from build123d import *

# Parameters (mm, degrees)
SKETCH1_R               = 25.65
SKETCH1_R_2             = 1.45
BOSS_EXTRUDE1_DEPTH     = 10
CUT_EXTRUDE2_DEPTH      = 38.627715849
CUT_EXTRUDE2_DEPTH_BACK = 7.4
SKETCH3_R               = 0.95
CUT_EXTRUDE3_DEPTH      = 10
BOSS_EXTRUDE2_DEPTH     = 41.5
BOSS_EXTRUDE3_REACH     = 72.472
SKETCH7_R               = 0.95
SKETCH7_W               = 10
SKETCH7_H               = 34.697559569
SKETCH11_R              = 0.95
CUT_EXTRUDE4_DEPTH      = 15


with BuildPart() as part:
    # Sketch1 → Boss-Extrude1 (new body)
    with BuildSketch(Plane.XY):
        Circle(SKETCH1_R)
        with Locations((0, -22.65)):
            Circle(SKETCH1_R_2, mode=Mode.SUBTRACT)
        with Locations((22.65, 0)):
            Circle(SKETCH1_R_2, mode=Mode.SUBTRACT)
        with Locations((0, 22.65)):
            Circle(SKETCH1_R_2, mode=Mode.SUBTRACT)
        with Locations((-22.65, 0)):
            Circle(SKETCH1_R_2, mode=Mode.SUBTRACT)
    extrude(amount=BOSS_EXTRUDE1_DEPTH)

    # Sketch2 → Cut-Extrude2 (cut, two sides: drawn at the far end of the back side and taken through both)
    with BuildSketch(Plane.XY.offset(10).offset(-CUT_EXTRUDE2_DEPTH_BACK)):
        Polygon((102.061719716, 116.734185426), (9.251139978, 23.923605688), (1.028840367, 15.701306076), (15.701306076, 1.028840367), (23.923605688, 9.251139978), (116.734185426, 102.061719716), (302.355344902, 287.682879192), (287.682879192, 302.355344902), align=None)
    extrude(amount=CUT_EXTRUDE2_DEPTH + CUT_EXTRUDE2_DEPTH_BACK, mode=Mode.SUBTRACT)

    # Sketch3 → Cut-Extrude3 (cut)
    with BuildSketch(Plane(origin=(8.365073221, 8.365073221, 0), x_dir=(0, 0, -1), z_dir=(0.7071067811865477, 0.7071067811865475, 0))):
        with Locations(Location((-5.74, 4.95, 0), (0, 0, 90))):
            Circle(SKETCH3_R)
        with Locations(Location((-5.74, -4.95, 0), (0, 0, 270))):
            Circle(SKETCH3_R)
    extrude(amount=-CUT_EXTRUDE3_DEPTH, mode=Mode.SUBTRACT)

    # Sketch5 → Boss-Extrude2 (add)
    with BuildSketch(Plane.XY.offset(10)):
        Polygon((15.701306076, 1.028840367), (5.693193293, -10.144237926), (10.907296496, -14.814690558), (20.915409279, -3.641612265), align=None)
        Polygon((0.245214439, 14.873396383), (-4.968888764, 19.543849015), (-14.977001547, 8.370770723), (-9.762898344, 3.700318091), align=None)
    extrude(amount=BOSS_EXTRUDE2_DEPTH)

    # Boss-Extrude3: up to this plane
    boss_extrude3_end = Plane(origin=(5.693193293, -10.144237926, 51.5), z_dir=(0.6672075188676077, 0.7448718861432019, 0))
    # Sketch7 → Boss-Extrude3 (add, up to the surface)
    with BuildSketch(Plane(origin=(8.365073221, 8.365073221, 0), x_dir=(0, 0, -1), z_dir=(0.7071067811865477, 0.7071067811865475, 0)), mode=Mode.PRIVATE) as boss_extrude3_sk1:
        with Locations((-5.74, -4.95)):
            Circle(SKETCH7_R)
    boss_extrude3_tool1 = split(extrude(boss_extrude3_sk1.sketch, amount=-BOSS_EXTRUDE3_REACH, mode=Mode.PRIVATE), bisect_by=boss_extrude3_end, keep=Keep.BOTH, mode=Mode.PRIVATE)
    add(boss_extrude3_tool1.solids().sort_by_distance((11.865252, 4.864895, 5.74))[0])
    # Sketch7 → Boss-Extrude3 (add, up to the surface)
    with BuildSketch(Plane(origin=(8.365073221, 8.365073221, 0), x_dir=(0, 0, -1), z_dir=(0.7071067811865477, 0.7071067811865475, 0)), mode=Mode.PRIVATE) as boss_extrude3_sk2:
        with Locations((-5.74, 4.95)):
            Circle(SKETCH7_R)
    boss_extrude3_tool2 = split(extrude(boss_extrude3_sk2.sketch, amount=-BOSS_EXTRUDE3_REACH, mode=Mode.PRIVATE), bisect_by=boss_extrude3_end, keep=Keep.BOTH, mode=Mode.PRIVATE)
    add(boss_extrude3_tool2.solids().sort_by_distance((4.864895, 11.865252, 5.74))[0])
    # Sketch7 → Boss-Extrude3 (add, up to the surface)
    with BuildSketch(Plane(origin=(8.365073221, 8.365073221, 0), x_dir=(0, 0, -1), z_dir=(0.7071067811865477, 0.7071067811865475, 0)), mode=Mode.PRIVATE) as boss_extrude3_sk3:
        with Locations((-56.5, -0.015656675)):
            Rectangle(SKETCH7_W, SKETCH7_H)
        with Locations(Location((-54.39, -4.95, 0), (0, 0, 270))):
            Circle(SKETCH7_R, mode=Mode.SUBTRACT)
        with Locations(Location((-54.39, 4.95, 0), (0, 0, 270))):
            Circle(SKETCH7_R, mode=Mode.SUBTRACT)
    boss_extrude3_tool3 = split(extrude(boss_extrude3_sk3.sketch, amount=-BOSS_EXTRUDE3_REACH, mode=Mode.PRIVATE), bisect_by=boss_extrude3_end, keep=Keep.BOTH, mode=Mode.PRIVATE)
    add(boss_extrude3_tool3.solids().sort_by_distance((8.376328, 8.353818, 56.535056))[0])

    # Sketch11 → Cut-Extrude4 (cut)
    with BuildSketch(Plane(origin=(8.365073221, 8.365073221, 0), x_dir=(0, 0, -1), z_dir=(0.7071067811865477, 0.7071067811865475, 0))):
        with Locations(Location((-5.74, -4.95, 0), (0, 0, 90))):
            Circle(SKETCH11_R)
        with Locations(Location((-5.74, 4.95, 0), (0, 0, 90))):
            Circle(SKETCH11_R)
    extrude(amount=-CUT_EXTRUDE4_DEPTH, mode=Mode.SUBTRACT)


solid = part.part
The model under review builds one solid part; all positions refer to its coordinate system, in mm. A direction names the side the tool comes from. Give positions to 0.01 mm unless a question says otherwise; leave off trailing zeros. Loops run counter-clockwise (first coordinate to the right, second up) from the corner with the lowest first, then second, coordinate; pieces in that order, holes last. Notation, with made-up numbers: (-17.75, -19) -> (32.25, -19) arc R16 ccw to (32.25, -11) -> close; hole circle Ø10 at (86.5, 8.25). An arc over 180 degrees is marked (long way). Answer as a JSON object with one key per item and string values. Group by question number.
Q1. Take a section at B-B (x = 22.65). Write out the cut boundary in (y, z), plus the area to 3 significant figures.
Q2. Take a section at D-D (x = 14.5). Write out the cut boundary in (y, z), plus the area to 3 significant figures.
Q3. Draft analysis for pull direction Z (two halves, no side actions). For faces 6 (the flat face through (12, 13, 2.6)), 7 (the flat face through (3, 3, 51.5)), 8 (the flat face through (-2.33, 17.18, 30.46)), 9 (the cylindrical face through (-0.189, 24.088, 4.93)), state which applies: pulls with the +Z half, pulls with the -Z half, needs draft (parallel to the pull), parting line crosses it, or undercut.
Q4. Take a section at A-A (z = 40). Write out the cut boundary in (x, y).
Q5. Insertion check: pin 1 (4 mm diameter, centred on x = 0, y = 22.65, fed in from -Z); pin 2 (10 mm diameter, centred on y = 4, z = 44, fed in from +X); pin 3 (2.5 mm diameter, centred on x = 0, y = -22.65, fed in from -Z); pin 4 (1 mm diameter, centred on x = 9.5, z = 16.5, fed in from +Y). Each pin has a flat end and moves straight along its axis. Give the tip position at first contact, or say it passes through.
Q6. Wall thickness on line 1 along Y through (x, z) = (0, 4.75); line 2 along Z through (x, y) = (-20, 11.5); line 3 along X through (y, z) = (-0.5, 7): over which ranges is each line inside the solid? List them lowest first.
Q7. Tool access review of faces 1 (the flat face through (-12, 12, 51.5)), 2 (the flat face through (8.26, 8.47, 6.35)), 3 (the flat face through (18.3, -1.3, 30.5)), 4 (the flat face through (15.541, -9.016, 56.57)), 5 (the flat face through (5.2, 19.87, 6.25)): name each direction out of +Z, -Z, +X, -X, +Y, -Y from which nothing blocks a thin tool from reaching the whole face with its end or side.
Answer below:
{
 "1": {"outline": "(-12.04, 0) -> (-1.45, 0) -> (-1.45, 10) -> (-12.04, 10) -> close; (1.45, 0) -> (12.04, 0) -> (12.04, 2.6) -> (7.98, 2.6) -> (7.98, 10) -> (1.45, 10) -> close", "area": "182 mm2"},
 "2": {"outline": "(-21.16, 0) -> (21.16, 0) -> (21.16, 2.6) -> (2.23, 2.6) -> (2.23, 10) -> (-0.31, 10) -> (-0.31, 51.5) -> (2.23, 51.5) -> (2.23, 61.5) -> (-10.06, 61.5) -> (-10.06, 51.5) -> (-10.8, 51.5) -> (-10.8, 10) -> (-21.16, 10) -> close", "area": "841 mm2"},
 "3": {"face 6": "pulls with the +Z half", "face 7": "undercut", "face 8": "undercut", "face 9": "needs draft"},
 "4": {"outline": "(-14.98, 8.37) -> (-9.76, 3.7) -> (0.25, 14.87) -> (-4.97, 19.54) -> close; (5.69, -10.14) -> (10.91, -14.81) -> (20.92, -3.64) -> (15.7, 1.03) -> close"},
 "5": {"pin 1": "stops at z = 0", "pin 2": "stops at x = 17.97", "pin 3": "passes through", "pin 4": "stops at y = -5.34"},
 "6": {"line 1": "y = -25.65 to -24.1, -21.2 to 21.2, 24.1 to 25.65", "line 2": "z = 0 to 10", "line 3": "x = -25.65 to -24.01, -21.29 to 21.29, 24.01 to 25.65"},
 "7": {"face 1": "-X, +Y", "face 2": "+Z", "face 3": "+Z, +X, +Y", "face 4": "+Z, +X, -Y", "face 5": "+Z, +X"}
}
